Model file for the job. Use its own axes, mm. A direction names the side the tool comes from. Round coordinates to 2 decimals unless told otherwise and drop trailing zeros. Write each loop counter-clockwise with the first axis right and the second up, starting at its lowest first coordinate (ties: lowest second). Pieces come first, ordered by that corner, then holes.
```python
from build123d import *

# Parameters (mm, degrees)
SKETCH1_R           = 40
BOSS_EXTRUDE1_DEPTH = 500
SKETCH2_R           = 30
CUT_EXTRUDE1_DEPTH  = 10
SKETCH3_R           = 35
CUT_EXTRUDE2_DEPTH  = 10


with BuildPart() as part:
    # Sketch1 → Boss-Extrude1 (new body)
    with BuildSketch(Plane.XY):
        Circle(SKETCH1_R)
    extrude(amount=BOSS_EXTRUDE1_DEPTH)

    # Sketch2 → Cut-Extrude1 (cut)
    with BuildSketch(Plane(origin=(0, 0, 500), x_dir=(-1, 0, 0), z_dir=(0, 0, -1))):
        Circle(SKETCH2_R)
    extrude(amount=CUT_EXTRUDE1_DEPTH, mode=Mode.SUBTRACT)

    # Sketch3 → Cut-Extrude2 (cut)
    with BuildSketch(Plane.XY.offset(490)):
        Circle(SKETCH3_R)
    extrude(amount=-CUT_EXTRUDE2_DEPTH, mode=Mode.SUBTRACT)


solid = part.part
```
1) Cut at A-A on y = 0. List the corners of the cut face in (x, z).
2) Cut at C-C on z = 260.5. List the corners of the cut face in (x, y), and give its area (3 significant figures).
3) Wall check: probe 1 along Y at (x, z) = (0, 482.5); probe 2 along Y at (x, z) = (0, 493); probe 3 along Z at (x, y) = (-21.5, -22). Give the ranges that are in metal, low to high.
4) Flat gauge pins, fed straight in: pin 1 Ø5 at (x, z) = (-19, 193) entering from +Y; pin 2 Ø1.5 at (x, z) = (-12.5, 394) entering from +Y; pin 3 Ø8 at (y, z) = (-5, 295) entering from +X. Where does each tip first touch, or does it go through?
5) Which spindle directions (+Z, -Z, +X, -X, +Y, -Y) get a long thin tool onto all of the face, cutting with end or side? Do faces 4 (the face through (0, 0, 480)), 5 (the face through (-1, 1, 0)), 6 (the face through (29.97, 1.32, 495.07)). Say none if no direction does.
6) Pull direction Z, two halves, no side cores. Call faces 1 (the face through (26, 16, 490)), 2 (the face through (6, 30, 500)), 3 (the face through (-8.67, -39.05, 246.5)): released by +Z, released by -Z, zero draft, split by the parting line, or undercut.
Result sheet:
1. outline: (-40, 0) - (40, 0) - (40, 500) - (30, 500) - (30, 490) - (35, 490) - (35, 480) - (-35, 480) - (-35, 490) - (-30, 490) - (-30, 500) - (-40, 500) - close
2. outline: circle Ø80 at (0, 0)
2. area: 5,030 mm2
3. probe 1: y = -40 to -35, 35 to 40
3. probe 2: y = -40 to -30, 30 to 40
3. probe 3: z = 0 to 480, 490 to 500
4. pin 1: stops at y = 36.44
4. pin 2: stops at y = 38.24
4. pin 3: stops at x = 39.99
5. face 4: none
5. face 5: -Z, +X, -X, +Y, -Y
5. face 6: +Z
6. face 1: undercut
6. face 2: released by +Z
6. face 3: zero draft
